Model file for the job. Use its own axes, mm. A direction names the side the tool comes from. Coordinates: 2 decimals unless noted, no trailing zeros. Order: outer loops, then holes, each group sorted by start corner. A loop starts at its lowest first (then second) coordinate and runs counter-clockwise, first axis right, second up. Notation, with made-up numbers: (60.25, -18.5) -> (100.25, -18.5) arc R25 cw to (100.25, 14.5) -> close; hole circle Ø11 at (52.5, 30). An arc over 180 degrees is marked (long way). Return JSON: item names as keys, results as strings. Group by question number.
1) Pull direction Z, two halves, no side cores. Call faces 1 (the flat face through (12, 62, 54.566)), 2 (the flat face through (34, 120, 56)), 3 (the flat face through (18, 59, -43.02)): +Z half, -Z half, draft (parallel to the pull), parting line (faces both ways), or undercut.
2) Which spindle directions (+Z, -Z, +X, -X, +Y, -Y) get a long thin tool onto all of the face, cutting with end or side? Do faces 4 (the flat face through (16, 0, 11)), 5 (the flat face through (84.666, 62, 10)). Say none if no direction does.
3) Probe line 1 (Z direction, x = -8, y = 69); line 2 (X direction, y = 28, z = -8); line 3 (Y direction, x = -15, z = -18). List the from-to ranges inside material, lowest first.
4) Cut at B-B (x = 61). Write the cut outline in (y, z).
5) Cut at A-A (y = 59.5). Write the cut outline in (x, z).
6) Cut at C-C (z = -25). Write the cut outline in (x, y).
7) Flat gauge pins, fed straight in: pin 1 (10 mm diameter, centred on x = 46.5, z = 37, fed in from +Y); pin 2 (1.5 mm diameter, centred on y = 32, z = 3.5, fed in from -X). Where does each tip first touch, or does it go through?
from build123d import *

# Parameters (mm, degrees)
BOSS_EXTRUDE1_DEPTH = 120
SKETCH2_W           = 158.061450485
SKETCH2_H           = 109.955791642
BOSS_EXTRUDE2_DEPTH = 5


with BuildPart() as part:
    # Sketch1 → Boss-Extrude1 (new body)
    with BuildSketch(Plane(origin=(0, 0, 0), x_dir=(1, 0, 0), z_dir=(0, 1, 0))):
        Polygon((-62.125022278, 33.67396119), (84.665959564, 33.67396119), (84.665959564, -54.565561602), (-62.125022278, -54.565561602), (-62.125022278, -66.935588162), (95.936428207, -66.935588162), (95.936428207, 43.02020348), (-62.125022278, 43.02020348), align=None)
    extrude(amount=BOSS_EXTRUDE1_DEPTH)

    # Sketch2 → Boss-Extrude2 (add)
    with BuildSketch(Plane.XZ):
        with Locations((16.905702965, 11.957692341)):
            Rectangle(SKETCH2_W, SKETCH2_H)
    extrude(amount=-BOSS_EXTRUDE2_DEPTH)


solid = part.part
Answers below:
{
 "1": {"face 1": "undercut", "face 2": "draft", "face 3": "-Z half"},
 "2": {"face 4": "+Z, -Z, +X, -X, -Y", "face 5": "-X, +Y"},
 "3": {"line 1": "z = -43.02 to -33.67, 54.57 to 66.94", "line 2": "x = 84.67 to 95.94", "line 3": "y = 0 to 5"},
 "4": {"outline": "(0, -43.02) -> (120, -43.02) -> (120, -33.67) -> (5, -33.67) -> (5, 54.57) -> (120, 54.57) -> (120, 66.94) -> (0, 66.94) -> close"},
 "5": {"outline": "(-62.13, -43.02) -> (95.94, -43.02) -> (95.94, 66.94) -> (-62.13, 66.94) -> (-62.13, 54.57) -> (84.67, 54.57) -> (84.67, -33.67) -> (-62.13, -33.67) -> close"},
 "6": {"outline": "(-62.13, 0) -> (95.94, 0) -> (95.94, 120) -> (84.67, 120) -> (84.67, 5) -> (-62.13, 5) -> close"},
 "7": {"pin 1": "stops at y = 5", "pin 2": "stops at x = 84.67"}
}
